Check sheet for the modelled part. Datum: model origin and axes. Units: mm. A direction names the side the tool comes from. Coordinates: 2 decimals unless noted, no trailing zeros. Write each loop counter-clockwise with the first axis right and the second up, starting at its lowest first coordinate (ties: lowest second). Pieces come first, ordered by that corner, then holes. Notation, with made-up numbers: M -37.5,0.25 L -26.5,0.25 A13 cw -26.5,10.25 Z; hole C 22,60.5 d1. An arc over 180 degrees is marked long. Answer as CSV lines item,"result".
Autodesk Inventor part; units mm, degrees
ref_plane "YZ Plane" through (0, 0, 0) normal (1, 0, 0) x (0, 1, 0)
ref_plane "XZ Plane" through (0, 0, 0) normal (0, 1, 0) x (-1, 0, 0)
ref_plane "XY Plane" through (0, 0, 0) normal (0, 0, 1) x (1, 0, 0)
sketch "Sketch1" plane through (0, 0, 0) normal (0, 0, 1) x (1, 0, 0)
  circle A0 centre (0, 0) radius 8
  dimension "d0" = 16
extrude "Extrusion1" add sketch "Sketch1" along normal blind 12
sketch "Sketch2" plane through (0, 0, 12) normal (0, 0, 1) x (1, 0, 0)
  circle A0 centre (0, 0) radius 8
  circle A1 centre (0, -8) radius 3
  circle A2 centre (0, 8) radius 3
  dimension "d3" = 6
  dimension "d4" = 6
extrude "Extrusion2" add sketch "Sketch2" against normal blind 8 contours A2 A0 | A0 A2 | A1 A0 | A0 A1
sketch "Sketch4" plane through (0, 0, 0) normal (1, 0, 0) x (0, 1, 0)
  line L0 (0, 0) -> (0, -2)
  arc A0 (-4.899, 0) -> (0, -2) centre (0, 5) ccw
  line L1 (0, 0) -> (-4.899, 0)
  point P0 (-7, 0)
  dimension "d10" = 2
revolve "Revolution1" add sketch "Sketch4" angle 360 about axis through (0, 0, 0) along (0, 0, -1)
fillet "Fillet2" radius 0.5 2 edges at (0, 11, 4) (0, -11, 4)
fillet "Fillet3" radius 1.5 1 edges at (-8, 0, 0)
sketch "Sketch6" plane through (0, 0, 12) normal (0, 0, 1) x (1, 0, 0)
  arc A0 (2.9468, 7.4375) -> (-2.9468, 7.4375) centre (0, 8) ccw
  circle A1 centre (0, 8) radius 1.25
  point P0 (0, 0)
  dimension "d16" = 2.5
extrude "Extrusion3" add sketch "Sketch6" along normal blind 1
fillet "Fillet4" radius 0.5 1 edges at (-1.25, 8, 13)
mirror "Mirror1" about plane through (0, 0, 0) normal (0, 1, 0) of "Extrusion3", "Fillet4"
properties part number "wheel3"
1) Thickness scan on line 1 along X through (y, z) = (8, 10); line 2 along Z through (x, y) = (-2.5, 5.5); line 3 along Y through (x, z) = (0.25, 3). Record the ranges inside material, lowest first.
Answer key:
line 1,"x = -3 to 3"
line 2,"z = 0 to 12"
line 3,"y = -8 to 8"
2) Section check A-A, the plane z = 3. Record the boundary of the cut face in (x, y), plus the area to 3 significant figures.
Answer key:
outline,"C 0,0 d16"
area,"201 mm2"
3) Section check B-B, the plane z = 6.5. Record the boundary of the cut face in (x, y), plus the area to 3 significant figures.
Answer key:
outline,"M -2.95,-7.44 A3 ccw long 2.95,-7.44 A8 ccw 2.95,7.44 A3 ccw long -2.95,7.44 A8 ccw Z"
area,"232 mm2"
4) Depth check by flat-ended pin: P1, Ø2.5, axis at x = 0.5, y = 8.5, coming from the -Z side; P2, Ø1.5, axis at y = -2, z = 5.5, coming from the +X side; P3, Ø5, axis at x = -1.5, y = 0, coming from the +Z side. Enter the tip coordinate at first touch or a pass-through.
Answer key:
P1,"stops at z = 0.21"
P2,"stops at x = 7.9"
P3,"stops at z = 12"
5) Tool access check on faces 1 (the face through (-0.27, -6.78, 12.25)), 2 (the face through (1, 5, 0)), 3 (the face through (0, 8, 13)). Record the directions out of +Z, -Z, +X, -X, +Y, -Y that give a thin tool (end or side, any length) a straight path to the whole face; none if there is none.
Answer key:
face 1,"+Z"
face 2,"-Z"
face 3,"+Z, +X, -X, +Y, -Y"
